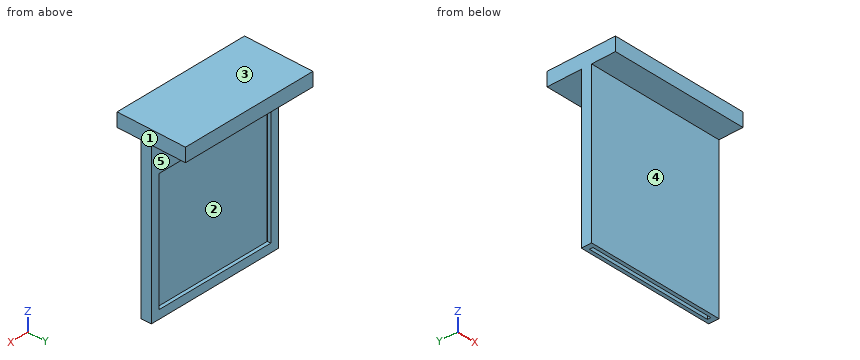
```python
from build123d import *

# Parameters (mm, degrees)
SKETCH1_W                = 8
SKETCH1_H                = 10
BOSS_EXTRUDE1_DEPTH      = 0.6
SKETCH4_W                = 7
SKETCH4_H                = 7
CUT_EXTRUDE1_DEPTH       = 0.4
SKETCH5_W                = 7.4
SKETCH5_H                = 0.2
CUT_EXTRUDE2_DEPTH       = 8
BOSS_EXTRUDE2_DEPTH      = 2
BOSS_EXTRUDE2_DEPTH_BACK = 2
SKETCH6_W                = 8
SKETCH6_H                = 0.8


with BuildPart() as part:
    # Sketch1 → Boss-Extrude1 (new body)
    with BuildSketch(Plane(origin=(0, 0, 0), x_dir=(1, 0, 0), z_dir=(0, 1, 0))):
        Rectangle(SKETCH1_W, SKETCH1_H)
    extrude(amount=BOSS_EXTRUDE1_DEPTH)

    # Sketch4 → Cut-Extrude1 (cut)
    with BuildSketch(Plane(origin=(0, 0.6, 0), x_dir=(1, 0, 0), z_dir=(0, 1, 0))):
        with Locations((0, 1)):
            Rectangle(SKETCH4_W, SKETCH4_H)
    extrude(amount=-CUT_EXTRUDE1_DEPTH, mode=Mode.SUBTRACT)

    # Sketch5 → Cut-Extrude2 (cut)
    with BuildSketch(Plane(origin=(0, 0, -5), x_dir=(-1, 0, 0), z_dir=(0, 0, -1))):
        with Locations((0, 0.3)):
            Rectangle(SKETCH5_W, SKETCH5_H)
    extrude(amount=-CUT_EXTRUDE2_DEPTH, mode=Mode.SUBTRACT)

    # Sketch6 → Boss-Extrude2 (add, two sides: drawn at the far end of the back side and taken through both)
    with BuildSketch(Plane(origin=(0, 0.6, 0), x_dir=(1, 0, 0), z_dir=(0, 1, 0)).offset(-BOSS_EXTRUDE2_DEPTH_BACK)):
        with Locations((0, -4.6)):
            Rectangle(SKETCH6_W, SKETCH6_H)
    extrude(amount=BOSS_EXTRUDE2_DEPTH + BOSS_EXTRUDE2_DEPTH_BACK)


solid = part.part
```
Work out the finished part from the listing and answer in its coordinate system (mm). Face numbers are marked on the shaded views. A direction names the side the tool comes from. Round coordinates to 2 decimals unless told otherwise and drop trailing zeros. Loops run counter-clockwise (first coordinate to the right, second up) from the corner with the lowest first, then second, coordinate; pieces in that order, holes last. Notation, with made-up numbers: M -21.5,19.25 L -14.5,19.25 A19 ccw -14.5,29.25 Z; hole C -19.75,58 d1. An arc over 180 degrees is marked long. Use CSV: the item, a comma, the result in double quotes.
Q1. Consider L1, parallel to X at y = 0.5, z = -3.5; L2, parallel to X at y = 0.35, z = 0.5; L3, parallel to Z at x = 2.5, y = -0.8. Determine where each line is inside the solid, lowest interval first.
Determined:
L1,"-4 to -3.5, 3.5 to 4"
L2,"-4 to -3.7, 3.7 to 4"
L3,"4.2 to 5"
Q2. Section A-A, the plane x = 0.75 is taken. Determine the outline of the cut face in (y, z), then the cut area to 3 significant figures.
Determined:
outline,"M -1.4,4.2 L 0,4.2 L 0,-5 L 0.2,-5 L 0.2,3 L 0.4,3 L 0.4,2.5 L 0.6,2.5 L 0.6,4.2 L 2.6,4.2 L 2.6,5 L -1.4,5 Z; M 0.4,-5 L 0.6,-5 L 0.6,-4.5 L 0.4,-4.5 Z"
area,"5.72 mm2"
Q3. Section D-D, the plane z = 3.75 is taken. Determine the outline of the cut face in (x, y), then the cut area to 3 significant figures.
Determined:
outline,"M -4,0 L 4,0 L 4,0.6 L -4,0.6 Z"
area,"4.80 mm2"
Q4. Section B-B, the plane z = -0.25 is taken. Determine the outline of the cut face in (x, y), then the cut area to 3 significant figures.
Determined:
outline,"M -4,0 L 4,0 L 4,0.6 L 3.5,0.6 L 3.5,0.4 L 3.7,0.4 L 3.7,0.2 L -3.7,0.2 L -3.7,0.4 L -3.5,0.4 L -3.5,0.6 L -4,0.6 Z"
area,"1.92 mm2"
Q5. The mould has two halves that part along X. Classify the marked faces 1, 2 and 3: pulls with the +X half, pulls with the -X half, needs draft (parallel to the pull), parting line crosses it, or undercut.
Determined:
face 1,"pulls with the +X half"
face 2,"undercut"
face 3,"needs draft"
Q6. Each of these flat-tipped pins is pushed along its axis until it touches: pin 1 (3 mm diameter, centred on x = -2.5, z = -4, fed in from -Y); pin 2 (0.6 mm diameter, centred on x = 2, y = 2, fed in from -Z); pin 3 (2.5 mm diameter, centred on x = 1.5, z = 1, fed in from +Y); pin 4 (1.5 mm diameter, centred on y = 2, z = 1, fed in from +X). Where does it stop, or does it pass through?
Determined:
pin 1,"y = 0"
pin 2,"z = 4.2"
pin 3,"y = 0.2"
pin 4,"through"
Q7. A tool of negligible diameter and unlimited length cuts with its end or side. For the marked faces 4 and 5, from which of +Z, -Z, +X, -X, +Y, -Y can it reach the whole face along a straight path? Write none if from no direction.
Determined:
face 4,"-Z, +X, -X, -Y"
face 5,"-Z, +X, -X, +Y"
Q8. Section C-C, the plane y = -0.4 is taken. Determine the outline of the cut face in (x, z).
Determined:
outline,"M -4,4.2 L 4,4.2 L 4,5 L -4,5 Z"
